Print and shaded views of the part. All mm, measured from the part's lowest x, y and z. A direction names the side the tool comes from. Round coordinates to 2 decimals unless told otherwise and drop trailing zeros. Order: outer loops, then holes, each group sorted by start corner. A loop starts at its lowest first (then second) coordinate and runs counter-clockwise, first axis right, second up. Notation, with made-up numbers: (16.25, 47) - (44.25, 47) arc R20 cw to (44.25, 59) - close; hole circle Ø6 at (64, 16.25). An arc over 180 degrees is marked (long way). Return JSON: item names as keys, results as strings. Group by question number.
Item 1: Drop flat-ended pins along their axis: pin 1 (3 mm diameter, centred on x = 20.5, z = 11.5, fed in from -Y); pin 2 (1.5 mm diameter, centred on x = 32, z = 11.5, fed in from +Y). Give the stop position or say it passes through.
Item 2: Saw through at B-B on z = 5.5. List the corners of the cut face in (x, y).
Item 3: Tool access for the marked faces 4 and 5: list every direction of +Z, -Z, +X, -X, +Y, -Y with a clear straight run to the whole face (end or side of a thin tool).
Item 4: Saw through at C-C on x = 33. List the corners of the cut face in (y, z), and give its area (3 significant figures).
Item 5: Probe probe 1 along Z at (x, y) = (21, 3.5); probe 2 along X at (y, z) = (2.8, 8.75); probe 3 along Y at (x, z) = (21.5, 3). List the from-to ranges inside material, lowest first.
Item 6: Two-plate mould, pull along X, no slides. Class the marked faces 1, 2 and 3: released by +X, released by -X, zero draft, split by the parting line, or undercut.
Item 7: Saw through at A-A on y = 3.4. List the corners of the cut face in (x, z).
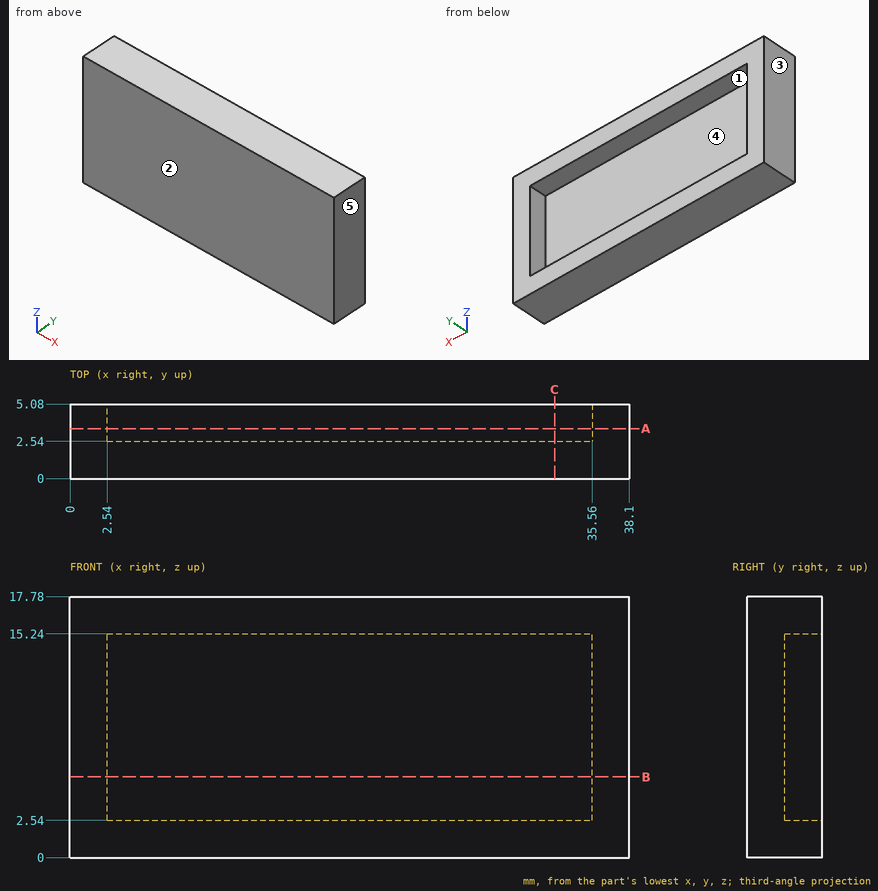
Filled in:
{
 "1": {"pin 1": "stops at y = 0", "pin 2": "stops at y = 2.54"},
 "2": {"outline": "(0, 0) - (38.1, 0) - (38.1, 5.08) - (35.56, 5.08) - (35.56, 2.54) - (2.54, 2.54) - (2.54, 5.08) - (0, 5.08) - close"},
 "3": {"face 4": "+Y", "face 5": "+Z, -Z, +X, +Y, -Y"},
 "4": {"outline": "(0, 0) - (5.08, 0) - (5.08, 2.54) - (2.54, 2.54) - (2.54, 15.24) - (5.08, 15.24) - (5.08, 17.78) - (0, 17.78) - close", "area": "58.1 mm^2"},
 "5": {"probe 1": "z = 0 to 2.54, 15.24 to 17.78", "probe 2": "x = 0 to 2.54, 35.56 to 38.1", "probe 3": "y = 0 to 2.54"},
 "6": {"face 1": "undercut", "face 2": "zero draft", "face 3": "released by -X"},
 "7": {"outline": "(0, 0) - (38.1, 0) - (38.1, 17.78) - (0, 17.78) - close; hole (2.54, 2.54) - (35.56, 2.54) - (35.56, 15.24) - (2.54, 15.24) - close"}
}
